```python
from build123d import *

# Parameters (mm, degrees)
SKETCH3_R               = 9.525
BOSS_EXTRUDE1_DEPTH     = 304.8
CHAMFER1_SIZE           = 1.42875
CUT_EXTRUDE1_START      = -101.6
CUT_EXTRUDE1_DEPTH      = 101.600004
CUT_EXTRUDE2_DEPTH      = 355.6
BOSS_EXTRUDE2_DEPTH     = 50.8
BOSS_EXTRUDE3_DEPTH     = 101.6
CUT_EXTRUDE3_DEPTH      = 306.153633722
CUT_EXTRUDE3_DEPTH_BACK = 306.153633722
SKETCH9_R               = 3.96875


with BuildPart() as part:
    # Sketch3 → Boss-Extrude1 (new, symmetric)
    with BuildSketch(Plane.XY):
        with Locations(Location((0, 0, 0), (0, 0, 180))):
            Circle(SKETCH3_R)
    extrude(amount=BOSS_EXTRUDE1_DEPTH, both=True)

    # Chamfer1
    chamfer1_edges = [part.edges().sort_by_distance(p)[0] for p in [
        (9.525, 0, -304.8),
        (9.525, 0, 304.8),
    ]]
    chamfer(chamfer1_edges, length=CHAMFER1_SIZE)

    # Sketch5 → Cut-Extrude1 (cut)
    with BuildSketch(Plane.XY.offset(304.8).offset(CUT_EXTRUDE1_START)):
        Polygon((-2.38125, 11.179201601), (2.38125, 11.179201601), (2.38125, 9.222541593), (2.38125, 6.841291593), (-2.38125, 6.841291593), (-2.38125, 9.222541593), align=None)
    extrude(amount=CUT_EXTRUDE1_DEPTH, mode=Mode.SUBTRACT)

    # Sketch6 → Cut-Extrude2 (cut)
    with BuildSketch(Plane(origin=(0, 0, -304.8), x_dir=(-1, 0, 0), z_dir=(0, 0, -1))):
        Polygon((2.38125, 11.179201601), (-2.38125, 11.179201601), (-2.38125, 9.222541593), (-2.38125, 6.841291593), (2.38125, 6.841291593), (2.38125, 9.222541593), align=None)
    extrude(amount=-CUT_EXTRUDE2_DEPTH, mode=Mode.SUBTRACT)

    # Sketch7 → Boss-Extrude2 (add)
    with BuildSketch(Plane.XY.offset(279.4)):
        Polygon((-2.38125, 11.179201601), (-2.38125, 9.222541593), (-2.38125, 6.841291593), (2.38125, 6.841291593), (2.38125, 9.222541593), (2.38125, 11.179201601), align=None)
    extrude(amount=-BOSS_EXTRUDE2_DEPTH)

    # Sketch8 → Boss-Extrude3 (add)
    with BuildSketch(Plane.XY.offset(-279.4)):
        Polygon((-2.38125, 11.179201601), (-2.38125, 9.222541593), (-2.38125, 6.841291593), (2.38125, 6.841291593), (2.38125, 9.222541593), (2.38125, 11.179201601), align=None)
    extrude(amount=BOSS_EXTRUDE3_DEPTH)

    # Sketch9 → Cut-Extrude3 (cut, two sides: drawn at the far end of the back side and taken through both)
    with BuildSketch(Plane(origin=(0, 0, 0), x_dir=(1, 0, 0), z_dir=(0, 1, 0)).offset(-CUT_EXTRUDE3_DEPTH_BACK)):
        with Locations(Location((0, 74.168, 0), (0, 0, 270))):
            Circle(SKETCH9_R)
    extrude(amount=CUT_EXTRUDE3_DEPTH + CUT_EXTRUDE3_DEPTH_BACK, mode=Mode.SUBTRACT)


solid = part.part
```
Geometry: final body of the model. Coordinates: model frame, mm. Give positions to 0.01 mm unless a question says otherwise; leave off trailing zeros. Order: outer loops, then holes, each group sorted by start corner. A loop starts at its lowest first (then second) coordinate and runs counter-clockwise, first axis right, second up. Notation, with made-up numbers: (61.5, 16) -> (82.5, 16) arc R33 ccw to (82.5, 49) -> close; hole circle Ø7 at (-27, -11). An arc over 180 degrees is marked (long way). Write each question's results on one line, items separated by ' | '. Start each with the question number.
1) Section B-B (z = -128). Return loops of the section in (x, y) (3 decimals), then the cut area to 3 significant figures.
2) Line query: line 1 (Z direction, x = -0.5, y = -5); line 2 (Z direction, x = -2.5, y = 5); line 3 (X direction, y = 1.5, z = -193.5). Output: solid intervals per line, ascending. Write a range as from..to.
3) Section A-A (z = 161). Return loops of the section in (x, y) (3 decimals), then the cut area to 3 significant figures.
4) First-contact query: pin 1 (1.2 mm diameter, centred on y = 7.5, z = 0, fed in from -X); pin 2 (1.2 mm diameter, centred on y = 8.5, z = 294.5, fed in from +X); pin 3 (1.2 mm diameter, centred on y = 8, z = -298, fed in from -X). Flat tips, straight axial feed; report the tip coordinate or a pass-through.
Calculated:
1) outline: (-2.381, 6.841) -> (-2.381, 9.223) arc R9.525 ccw (long way) to (2.381, 9.223) -> (2.381, 6.841) -> close | area: 273 mm2
2) line 1: -304.8..-78.11, -70.23..304.8 | line 2: -304.8..-77.25, -71.09..304.8 | line 3: -9.41..9.41
3) outline: circle Ø19.05 at (0, 0) | area: 285 mm2
4) pin 1: x = -6.57 | pin 2: x = 5.32 | pin 3: x = -6
